The model under review builds one solid part; all positions refer to its coordinate system, in mm. A direction names the side the tool comes from. Coordinates: 2 decimals unless noted, no trailing zeros. Write each loop counter-clockwise with the first axis right and the second up, starting at its lowest first coordinate (ties: lowest second). Pieces come first, ordered by that corner, then holes. Notation, with made-up numbers: (-19.5, -34) - (0.5, -34) arc R18 ccw to (0.5, -19) - close; hole circle Ø5 at (20, -25). An arc over 180 degrees is marked (long way). Return JSON: item names as keys, results as strings. Group by question number.
(1) We need section D-D on z = 23. State the section outline as (x, y) points.
(2) To check wall thickness, follow L1, parallel to Z at x = 0, y = 3 (1 decimal); L2, parallel to Y at x = -1.25, z = 12; L3, parallel to Z at x = -1.75, y = -3.75. State the ranges of each line that lie inside material, in increasing order. Write a range as from..to.
(3) For pin 1 Ø2 at (y, z) = (2.5, 45.5) entering from +X; pin 2 Ø3 at (x, z) = (0, 26.5) entering from +Y; pin 3 Ø1.5 at (y, z) = (-0.5, 17.5) entering from -X, all flat-tipped, find the tip position at first contact; note any pin that passes through.
(4) We need section B-B on x = -2.5. State the section outline as (y, z) points.
(5) Tool access review of faces 1 (the face through (-0.21, -4, 3.17)), 2 (the face through (-0.34, 0.09, -1.55)), 3 (the face through (-0.21, 3.94, 3.17)): name each direction out of +Z, -Z, +X, -X, +Y, -Y from which nothing blocks a thin tool from reaching the whole face with its end or side.
```python
from build123d import *

# Parameters (mm, degrees)
F0_R     = 1.5875
F1_DEPTH = 6.35
F2_DEPTH = 1.5875


with BuildPart() as f1:
    # F0 (on Front) → F1 (new body, symmetric)
    with BuildSketch(Plane.XZ):
        with BuildLine():
            ThreePointArc((-3.1749141346, 0.0233503235), (-0.2706319367, -3.1634448557), (3.1327451143, -0.5162683885))
            Line((3.1327451143, -0.5162683885), (3.0466813259, 0.8935087569))
            ThreePointArc((3.0466813259, 0.8935087569), (-0.2659699045, 3.1638402314), (-3.153094005, 0.3723213606))
            Line((-3.153094005, 0.3723213606), (-3.1749141346, 0.0233503235))
        make_face()
        Circle(F0_R, mode=Mode.SUBTRACT)
    extrude(amount=F1_DEPTH, both=True)

    # F0 (on Front) → F2 (join, symmetric)
    with BuildSketch(Plane.XZ):
        with BuildLine():
            ThreePointArc((-3.153094005, 0.3723213606), (-0.2659699045, 3.1638402314), (3.0466813259, 0.8935087569))
            Line((3.0466813259, 0.8935087569), (0, 50.8))
            Line((0, 50.8), (-3.153094005, 0.3723213606))
        make_face()
    extrude(amount=F2_DEPTH, both=True)


solid = f1.part
```
Ans:
{
 "1": {"outline": "(-1.74, -1.59) - (1.7, -1.59) - (1.7, 1.59) - (-1.74, 1.59) - close"},
 "2": {"L1": "-3.2..-1.6, 1.6..3.2", "L2": "-1.59..1.59", "L3": "-2.65..2.65"},
 "3": {"pin 1": "x = 0.35", "pin 2": "y = 1.59", "pin 3": "x = -2.13"},
 "4": {"outline": "(-6.35, -1.96) - (6.35, -1.96) - (6.35, 1.96) - (1.59, 1.96) - (1.59, 10.82) - (-1.59, 10.82) - (-1.59, 1.96) - (-6.35, 1.96) - close"},
 "5": {"face 1": "+Z, -Y", "face 2": "+Y, -Y", "face 3": "+Z, +Y"}
}
